from build123d import *

# Parameters (mm, degrees)
F0_W     = 76.2
F0_H     = 127
F1_DEPTH = 25.4
F2_R     = 5.08
F3_W     = 25.4
F3_H     = 76.2
F4_DEPTH = 12.7
F5_R     = 5.08


with BuildPart() as f1:
    # F0 (on Top) → F1 (new body)
    with BuildSketch(Plane.XY):
        with Locations((38.1, -63.5)):
            Rectangle(F0_W, F0_H)
    extrude(amount=F1_DEPTH)

    # F2
    f2_edges = [f1.edges().sort_by_distance(p)[0] for p in [
        (0, -127, 12.7),
        (76.2, -127, 12.7),
    ]]
    fillet(f2_edges, radius=F2_R)

    # F3 (on face) → F4 (cut)
    with BuildSketch(Plane.XY.offset(25.4)):
        with Locations((38.1, -63.5)):
            Rectangle(F3_W, F3_H)
    extrude(amount=-F4_DEPTH, mode=Mode.SUBTRACT)

    # F5
    f5_edges = [f1.edges().sort_by_distance(p)[0] for p in [
        (50.8, -25.4, 19.05),
        (25.4, -25.4, 19.05),
        (50.8, -101.6, 19.05),
        (25.4, -101.6, 19.05),
    ]]
    fillet(f5_edges, radius=F5_R)


solid = f1.part
Here's how the part is built. I have some questions about the finished solid (model axes, mm). A direction names the side the tool comes from. Give positions to 0.01 mm unless a question says otherwise; leave off trailing zeros. Loops run counter-clockwise (first coordinate to the right, second up) from the corner with the lowest first, then second, coordinate; pieces in that order, holes last. Notation, with made-up numbers: (7.5, -31) -> (30.5, -31) arc R15 cw to (30.5, -11) -> close; hole circle Ø11 at (-6.5, 73). An arc over 180 degrees is marked (long way). Answer as a JSON object with one key per item and string values. Group by question number.
Item 1: Imagine slicing it at A-A on y = -50.5. Write out the boundary of the cut face in (x, z).
Item 2: Imagine slicing it at C-C on x = 34. Write out the boundary of the cut face in (y, z).
Item 3: Thinking about a two-plate mould opening in X: for faces 1 (the flat face through (76.2, -62, 13)), 2 (the flat face through (38, -63, 12.7)), 3 (the flat face through (54, -63, 25.4)), which applies, pulls with the +X half, pulls with the -X half, needs draft (parallel to the pull), parting line crosses it, or undercut?
Item 4: On a 3-axis mill with a long thin cutter (end or side, diameter ignored), from which of +Z, -Z, +X, -X, +Y, -Y can I reach the whole of each face in a straight line? I mean faces 4 (the cylindrical face through (74.672, -125.551, 12.878)), 5 (the flat face through (38, -101.6, 19)). Say none if no direction works.
Item 5: I need wall thicknesses on L1, parallel to X at y = -68, z = 24.25; L2, parallel to Y at x = 5, z = 1.25; L3, parallel to X at y = -26, z = 21.5 (3 decimals). Which ranges of each line are inside material? Lowest first, please.
Item 6: Imagine slicing it at B-B on z = 18.75. Write out the boundary of the cut face in (x, y).
Item 7: Will this pin go through, and if not, where does the flat tip stop? pin 1 (12 mm diameter, centred on x = 57, y = -108, fed in from -Z).
Answer list:
{
 "1": {"outline": "(0, 0) -> (76.2, 0) -> (76.2, 25.4) -> (50.8, 25.4) -> (50.8, 12.7) -> (25.4, 12.7) -> (25.4, 25.4) -> (0, 25.4) -> close"},
 "2": {"outline": "(-127, 0) -> (0, 0) -> (0, 25.4) -> (-25.4, 25.4) -> (-25.4, 12.7) -> (-101.6, 12.7) -> (-101.6, 25.4) -> (-127, 25.4) -> close"},
 "3": {"face 1": "pulls with the +X half", "face 2": "undercut", "face 3": "needs draft"},
 "4": {"face 4": "+Z, -Z, +X, -Y", "face 5": "+Z"},
 "5": {"L1": "x = 0 to 25.4, 50.8 to 76.2", "L2": "y = -127 to 0", "L3": "x = 0 to 28.085, 48.115 to 76.2"},
 "6": {"outline": "(0, -121.92) arc R5.08 ccw to (5.08, -127) -> (71.12, -127) arc R5.08 ccw to (76.2, -121.92) -> (76.2, 0) -> (0, 0) -> close; hole (25.4, -96.52) arc R5.08 ccw to (30.48, -101.6) -> (45.72, -101.6) arc R5.08 ccw to (50.8, -96.52) -> (50.8, -30.48) arc R5.08 ccw to (45.72, -25.4) -> (30.48, -25.4) arc R5.08 ccw to (25.4, -30.48) -> close"},
 "7": {"pin 1": "stops at z = 0"}
}
